The model under review builds one solid part; all positions refer to its coordinate system, in mm. A direction names the side the tool comes from. Coordinates: 2 decimals unless noted, no trailing zeros. Order: outer loops, then holes, each group sorted by start corner. A loop starts at its lowest first (then second) coordinate and runs counter-clockwise, first axis right, second up. Notation, with made-up numbers: M -34.75,11 L 13.25,11 A14 ccw 13.25,31 Z; hole C 47.5,69.25 d3. An arc over 180 degrees is marked long. Answer in a Markdown table with one row per item.
from build123d import *

# Parameters (mm, degrees)
F0_W     = 1392
F0_H     = 188
F1_DEPTH = 450
F2_SIZE  = 2


# Not quite as in the source:
# - a feature names something its author has since deleted; it is built from what else it names


with BuildPart() as f1:
    # F0 (on Front) → F1 (new body)
    with BuildSketch(Plane.XZ):
        Polygon((750, 250), (-750, 250), (-750, -250), (600, -250), (600, -196), (-696, -196), (-696, -46), (750, -46), align=None)
        with Locations((0, 102)):
            Rectangle(F0_W, F0_H, mode=Mode.SUBTRACT)
    extrude(amount=F1_DEPTH)

    # F2
    f2_edges = [f1.edges().sort_by_distance(p)[0] for p in [
        (-750, -225, 250),
        (-750, -225, -250),
        (-750, 0, 0),
        (-750, -450, 0),
        (750, -225, 250),
        (0, 0, 250),
        (0, -450, 250),
        (750, -225, -46),
        (750, 0, 102),
        (750, -450, 102),
        (-75, -450, -250),
        (600, -450, -223),
        (-48, -450, -196),
        (-696, -450, -121),
        (27, -450, -46),
        (-696, -450, 102),
        (0, -450, 196),
        (696, -450, 102),
        (0, -450, 8),
        (-75, 0, -250),
        (600, 0, -223),
        (-48, 0, -196),
        (-696, 0, -121),
        (27, 0, -46),
        (-696, 0, 102),
        (0, 0, 196),
        (696, 0, 102),
        (0, 0, 8),
        (600, -225, -196),
    ]]
    chamfer(f2_edges, length=F2_SIZE)


solid = f1.part
(1) To check wall thickness, follow line 1 (Z direction, x = 1, y = -414); line 2 (X direction, y = -292.5, z = 133); line 3 (X direction, y = -82.5, z = -99). State the ranges of each line that lie inside material, in increasing order. Write a range as [from, to].
Report:
| item | result |
|---|---|
| line 1 | [-250, -196], [-46, 8], [196, 250] |
| line 2 | [-750, -696], [696, 750] |
| line 3 | [-750, -696] |
(2) Take a section at A-A (x = -412). Write out the cut boundary in (y, z), then the cut area to 3 significant figures.
Report:
| item | result |
|---|---|
| outline | M -450,-248 L -448,-250 L -2,-250 L 0,-248 L 0,-198 L -2,-196 L -448,-196 L -450,-198 Z; M -450,-44 L -448,-46 L -2,-46 L 0,-44 L 0,6 L -2,8 L -448,8 L -450,6 Z; M -450,198 L -448,196 L -2,196 L 0,198 L 0,248 L -2,250 L -448,250 L -450,248 Z |
| area | 72,900 mm^2 |
(3) Take a section at B-B (y = -97). Write out the cut boundary in (x, z).
Report:
| item | result |
|---|---|
| outline | M -750,-248 L -748,-250 L 600,-250 L 600,-198 L 598,-196 L -696,-196 L -696,-46 L 748,-46 L 750,-44 L 750,248 L 748,250 L -748,250 L -750,248 Z; hole M -696,8 L 696,8 L 696,196 L -696,196 Z |
(4) Take a section at D-D (z = -94). Write out the cut boundary in (x, y), then the cut area to 3 significant figures.
Report:
| item | result |
|---|---|
| outline | M -750,-448 L -748,-450 L -698,-450 L -696,-448 L -696,-2 L -698,0 L -748,0 L -750,-2 Z |
| area | 24,300 mm^2 |
(5) Take a section at C-C (z = 74.5). Write out the cut boundary in (x, y), then the cut area to 3 significant figures.
Report:
| item | result |
|---|---|
| outline | M -750,-448 L -748,-450 L -698,-450 L -696,-448 L -696,-2 L -698,0 L -748,0 L -750,-2 Z; M 696,-448 L 698,-450 L 748,-450 L 750,-448 L 750,-2 L 748,0 L 698,0 L 696,-2 Z |
| area | 48,600 mm^2 |
(6) The part is to be moulded in two halves that separate along X. For faces 1 (the flat face through (-750, -222, 3)), 2 (the flat face through (-83, -222, -250)), 3 (the flat face through (-10, -222, 196)), 4 (the flat face through (750, -222, 100)), say which applies: +X half, -X half, draft (parallel to the pull), parting line (faces both ways), or undercut.
Report:
| item | result |
|---|---|
| face 1 | -X half |
| face 2 | draft |
| face 3 | undercut |
| face 4 | +X half |
(7) Machinability: for faces 5 (the flat face through (-59, -450, 1)), 6 (the flat face through (-10, -222, 8)), 7 (the flat face through (-40, -222, -196)), 8 (the flat face through (600, -222, -224)), 9 (the flat face through (-59, 0, 1)), which of the approach directions +Z, -Z, +X, -X, +Y, -Y give a long, thin tool a straight path to every point of the face, cutting with its end or side? Answer none if there is none.
Report:
| item | result |
|---|---|
| face 5 | +Z, -Z, +X, -X, -Y |
| face 6 | +Y, -Y |
| face 7 | +X, +Y, -Y |
| face 8 | -Z, +X, +Y, -Y |
| face 9 | +Z, -Z, +X, -X, +Y |
(8) Insertion check: P1, Ø6, axis at y = -149, z = -77.5, coming from the +X side. The pin has a flat end and moves straight along its axis. Give the tip position at first contact, or say it passes through.
Report:
| item | result |
|---|---|
| P1 | x = -696 |
